from build123d import *

# Parameters (mm, degrees)
CROQUIS1_R                 = 12.5
SALIENTE_EXTRUIR1_DEPTH    = 165
CROQUIS2_R                 = 11.5
CORTAR_EXTRUIR1_DEPTH      = 166
EXTRUIR_L_MINA1_DEPTH      = 20
CORTAR_EXTRUIR4_DEPTH      = 5
CORTAR_EXTRUIR4_DEPTH_BACK = 34
CROQUIS6_R                 = 2.999725426
CORTAR_EXTRUIR5_DEPTH      = 5


with BuildPart() as part:
    # Croquis1 → Saliente-Extruir1 (new body)
    with BuildSketch(Plane(origin=(0, 0, 0), x_dir=(1, 0, 0), z_dir=(0, 1, 0))):
        Circle(CROQUIS1_R)
    extrude(amount=SALIENTE_EXTRUIR1_DEPTH)

    # Croquis2 → Cortar-Extruir1 (cut, through all)
    with BuildSketch(Plane(origin=(0, 165, 0), x_dir=(1, 0, 0), z_dir=(0, 1, 0))):
        Circle(CROQUIS2_R)
    extrude(amount=-CORTAR_EXTRUIR1_DEPTH, mode=Mode.SUBTRACT)

    # Croquis4 → Extruir-Lámina1 (add)
    with BuildSketch(Plane.XY):
        Polygon((-14.5, -69.456832295), (-14.5, -44.456832295), (-18.5, -30), (-18.5, 0), (18.5, 0), (18.5, -30), (14.5, -44.456832295), (14.5, -69.456832295), (13.5, -69.456832295), (13.5, -44.321040369), (17.5, -29.864208074), (17.5, -1), (-17.5, -1), (-17.5, -29.864208074), (-13.5, -44.321040369), (-13.5, -69.456832295), align=None)
    extruir_l_mina1 = extrude(amount=EXTRUIR_L_MINA1_DEPTH)

    # Simetría1: Extruir-Lámina1 across plane
    add(extruir_l_mina1.mirror(Plane.XY))

    # Croquis5 → Cortar-Extruir4 (cut, two sides)
    with BuildSketch(Plane.ZY.offset(14.5)) as cortar_extruir4_sk:
        Polygon((20, -23), (11.165079241, -44.456832295), (20, -44.456832295), align=None)
        with BuildLine():
            Line((20, -44.456832295), (11.165079241, -44.456832295))
            Line((11.165079241, -44.456832295), (4.058522787, -61.716091794))
            ThreePointArc((4.058522787, -61.716091794), (-0.338082334, -67.201681505), (-7, -69.446828292))
            Line((-7, -69.446828292), (-7, -69.456832295))
            Line((-7, -69.456832295), (20, -69.456832295))
            Line((20, -69.456832295), (20, -44.456832295))
        make_face()
        with BuildLine():
            Line((-19.747448714, -59.456832295), (-20, -59.456832295))
            Line((-20, -59.456832295), (-20, -69.456832295))
            Line((-20, -69.456832295), (-7.500000063, -69.456832295))
            ThreePointArc((-7.500000063, -69.456832295), (-15.405694175, -66.63929064), (-19.747448714, -59.456832295))
        make_face()
        with BuildLine():
            ThreePointArc((-2, -59.456832295), (-7, -54.456832295), (-12, -59.456832295))
            Line((-12, -59.456832295), (-7, -59.456832295))
            Line((-7, -59.456832295), (-7, -64.456832295))
            ThreePointArc((-7, -64.456832295), (-3.464466094, -62.992366201), (-2, -59.456832295))
        make_face()
        with BuildLine():
            Line((-7, -59.456832295), (-12, -59.456832295))
            ThreePointArc((-12, -59.456832295), (-10.535533906, -62.992366201), (-7, -64.456832295))
            Line((-7, -64.456832295), (-7, -59.456832295))
        make_face()
    extrude(amount=CORTAR_EXTRUIR4_DEPTH, mode=Mode.SUBTRACT)
    extrude(cortar_extruir4_sk.sketch, amount=-CORTAR_EXTRUIR4_DEPTH_BACK, mode=Mode.SUBTRACT)

    # Croquis6 → Cortar-Extruir5 (cut, symmetric)
    with BuildSketch(Plane(origin=(-0.184914892, 0, -12.485243343), x_dir=(-0.99989034, 0, 0.014809052), z_dir=(-0.014809052, 0, -0.99989034))):
        with Locations((0.848128323, 108.600309026)):
            Circle(CROQUIS6_R)
    extrude(amount=CORTAR_EXTRUIR5_DEPTH, both=True, mode=Mode.SUBTRACT)


solid = part.part
Can you work these out from the model? Positions are in its coordinate system, mm. A direction names the side the tool comes from. Round coordinates to 2 decimals unless told otherwise and drop trailing zeros. Loops run counter-clockwise (first coordinate to the right, second up) from the corner with the lowest first, then second, coordinate; pieces in that order, holes last. Notation, with made-up numbers: (52, 51) - (107, 51) arc R20 cw to (107, 63) - close; hole circle Ø1 at (72, 24). An arc over 180 degrees is marked (long way). Use CSV: the item, a comma, the result in double quotes. Start each with the question number.
1) Please list where these lines run through material, in increasing order: probe 1 along X at (y, z) = (58, 0); probe 2 along X at (y, z) = (-2, -17.5). Write a range as [from, to].
2) For faces 4 (the flat face through (-15.53, -36.99, -1.15)), 5 (the flat face through (-13, 0, 0)), 6 (the flat face through (14.5, -54, -8)), 7 (the flat face through (-14.5, -54, -8)), which set-ups out of +Z, -Z, +X, -X, +Y, -Y let a thin tool reach every point of the face, with its end or its side?
3) If we section it at C-C on x = 8: Write out the boundary of the cut face in (y, z), plus the area to 3 significant figures.
4) If we section it at B-B on z = 0: Write out the boundary of the cut face in (x, y).
5) If we section it at A-A on y = 99: Write out the boundary of the cut face in (x, z).
6) For pin 1 Ø1 at (x, z) = (-1.5, 9.5) entering from -Y; pin 2 Ø1 at (x, z) = (-13.5, -10.5) entering from -Y; pin 3 Ø20 at (y, z) = (-60, -8.5) entering from +X; pin 4 Ø5 at (x, z) = (5.5, -9.5) entering from +Y, each with a flat end and sliding along its axis, tell me the tip position at first contact or that it passes through.
7) We'd pull the mould along Z, two halves only. Please class faces 1 (the cylindrical face through (13.993, -67.144, -0.257)), 2 (the flat face through (13.5, -54, -8)), 3 (the cylindrical face through (-1.5, 83.7, -11.4)): released by +Z, released by -Z, zero draft, split by the parting line, or undercut.
Geometry results:
1,probe 1,"x = [-12.5, -11.5], [11.5, 12.5]"
1,probe 2,"x = [-18.5, -17.5], [17.5, 18.5]"
2,face 4,"+Z, -Z"
2,face 5,"+Y"
2,face 6,"+Z, -Z, +X, -Y"
2,face 7,"+Z, -Z, -X, -Y"
3,outline,"(-1, -20) - (0, -20) - (0, -9.6) - (165, -9.6) - (165, -8.26) - (0, -8.26) - (0, 8.26) - (165, 8.26) - (165, 9.6) - (0, 9.6) - (0, 20) - (-1, 20) - close"
3,area,"483 mm2"
4,outline,"(-18.5, -30) - (-14.5, -44.46) - (-14.5, -66.96) - (-13.5, -66.96) - (-13.5, -44.32) - (-17.5, -29.86) - (-17.5, -1) - (17.5, -1) - (17.5, -29.86) - (13.5, -44.32) - (13.5, -66.96) - (14.5, -66.96) - (14.5, -44.46) - (18.5, -30) - (18.5, 0) - (12.5, 0) - (12.5, 165) - (11.5, 165) - (11.5, 0) - (-11.5, 0) - (-11.5, 165) - (-12.5, 165) - (-12.5, 0) - (-18.5, 0) - close"
5,outline,"circle Ø25 at (0, 0); hole circle Ø23 at (0, 0)"
6,pin 1,"stops at y = -1"
6,pin 2,"stops at y = -69.2"
6,pin 3,"stops at x = 14.5"
6,pin 4,"stops at y = 165"
7,face 1,"released by +Z"
7,face 2,"zero draft"
7,face 3,"undercut"
